Geometry check sheet. Reference: the model listing, model coordinates, mm. Give positions to 0.01 mm unless a question says otherwise; leave off trailing zeros. Loops run counter-clockwise (first coordinate to the right, second up) from the corner with the lowest first, then second, coordinate; pieces in that order, holes last. Notation, with made-up numbers: (3, 44) -> (29, 44) arc R33 ccw to (29, 77) -> close; hole circle Ø4 at (8.25, -24.5). An arc over 180 degrees is marked (long way). One line per item, written item: value. Start each with the question number.
(1) Sectioned sample at A-A, the plane y = 0. Record the cut outline in (x, z), then the cut area to 3 significant figures.
(2) Scan lines: line 1 along X through (y, z) = (-2, 2.4); line 2 along X through (y, z) = (1, 0.25); line 3 along X through (y, z) = (3.5, 1.85). Record each from-to range of solid material in increasing order. Write a range as from..to.
(3) Draft check along Y on faces 1 (the face through (-0.192, -26.037, 1.252)), 2 (the face through (-10.19, 45.87, 1.25)), 3 (the face through (0, -28, 0)). Enter one of: pulls with the +Y half, pulls with the -Y half, needs draft (parallel to the pull), parting line crosses it, or undercut.
(4) Sectioned sample at D-D, the plane y = -40.64. Record the cut outline in (x, z).
(5) Sectioned sample at C-C, the plane z = 1.2. Record the cut outline in (x, y).
(6) Sectioned sample at B-B, the plane x = 0. Record the cut outline in (y, z).
(7) Gauge pin test, flat ends, axial feed: pin 1 Ø1.5 at (x, z) = (-16, 1) entering from +Y; pin 2 Ø4.5 at (x, y) = (0, 40.64) entering from -Z; pin 3 Ø1.5 at (x, z) = (24, 1.5) entering from +Y (3 decimals). Record the tip position at first contact, or that the pin passes through.
Autodesk Inventor part; units mm, degrees
ref_plane "YZ Plane" through (0, 0, 0) normal (1, 0, 0) x (0, 1, 0)
ref_plane "XZ Plane" through (0, 0, 0) normal (0, 1, 0) x (-1, 0, 0)
ref_plane "XY Plane" through (0, 0, 0) normal (0, 0, 1) x (1, 0, 0)
sketch "Sketch1" plane through (0, 0, 0) normal (0, 0, 1) x (1, 0, 0)
  arc A0 (9.4392, -34.2843) -> (-9.4392, -34.2843) centre (0, 0) ccw
  circle A1 centre (0, 0) radius 46.99
  arc A2 (9.4392, -34.2843) -> (-9.4392, -34.2843) centre (0, -35.56) ccw
  circle A3 centre (0, 40.64) radius 2.5527
  circle A4 centre (-40.64, 0) radius 2.5527
  circle A5 centre (0, -40.64) radius 2.5527
  circle A6 centre (40.64, 0) radius 2.5527
  point P0 (0, 46.99)
  dimension "d1" = 93.98
  dimension "d0" = 71.12
  dimension "d2" = 19.05
  dimension "d8" = 360
  dimension "d12" = 5.1054
  dimension "d13" = 6.35
extrude "Extrusion1" add sketch "Sketch1" along normal blind 2.54
properties part number "Gasket" material "Aluminum 6061"
Calculated:
1. outline: (-46.99, 0) -> (-43.19, 0) -> (-43.19, 2.54) -> (-46.99, 2.54) -> close; (-38.09, 0) -> (-35.56, 0) -> (-35.56, 2.54) -> (-38.09, 2.54) -> close; (35.56, 0) -> (38.09, 0) -> (38.09, 2.54) -> (35.56, 2.54) -> close; (43.19, 0) -> (46.99, 0) -> (46.99, 2.54) -> (43.19, 2.54) -> close
1. area: 32.1 mm2
2. line 1: x = -46.95..-42.23, -39.05..-35.5, 35.5..39.05, 42.23..46.95
2. line 2: x = -46.98..-42.99, -38.29..-35.55, 35.55..38.29, 42.99..46.98
2. line 3: x = -46.86..-35.39, 35.39..46.86
3. face 1: undercut
3. face 2: parting line crosses it
3. face 3: needs draft
4. outline: (-23.59, 0) -> (-2.55, 0) -> (-2.55, 2.54) -> (-23.59, 2.54) -> close; (2.55, 0) -> (23.59, 0) -> (23.59, 2.54) -> (2.55, 2.54) -> close
5. outline: circle Ø93.98 at (0, 0); hole circle Ø5.11 at (-40.64, 0); hole (-9.44, -34.28) arc R9.53 cw to (9.44, -34.28) arc R35.56 ccw (long way) to start; hole circle Ø5.11 at (0, -40.64); hole circle Ø5.11 at (0, 40.64); hole circle Ø5.11 at (40.64, 0)
6. outline: (-46.99, 0) -> (-43.19, 0) -> (-43.19, 2.54) -> (-46.99, 2.54) -> close; (-38.09, 0) -> (-26.03, 0) -> (-26.03, 2.54) -> (-38.09, 2.54) -> close; (35.56, 0) -> (38.09, 0) -> (38.09, 2.54) -> (35.56, 2.54) -> close; (43.19, 0) -> (46.99, 0) -> (46.99, 2.54) -> (43.19, 2.54) -> close
7. pin 1: stops at y = 44.45
7. pin 2: passes through
7. pin 3: stops at y = 40.835
